Input: part model. Units: mm. Frame: model coordinates. A direction names the side the tool comes from. Coordinates: 2 decimals unless noted, no trailing zeros. Order: outer loops, then holes, each group sorted by start corner. A loop starts at its lowest first (then second) coordinate and runs counter-clockwise, first axis right, second up. Notation, with made-up numbers: M 7.25,84.25 L 38.25,84.25 A22 cw 38.25,110.25 Z; hole C 69.25,74 d11. An arc over 180 degrees is marked long. One line per item, written item: value.
```python
from build123d import *

# Parameters (mm, degrees)
SKETCH_1_R                   = 6.5
EXTRUDE_1_DEPTH              = 6.5
CUT_EXTRUDE_1_DEPTH          = 37.704904304
FILLET_2_R                   = 2.3
SWEEP_START                  = -22.062157242
SWEEP_2_DEPTH                = 13.492384883
CHAMFER_1_SIZE               = 0.5
FILLET_3_R                   = 3
HOLE_WIZARD_M2_1_D           = 2.4
HOLE_WIZARD_M2_1_DEPTH       = 8.5
HOLE_WIZARD_M2_1_CBORE_D     = 4.1
HOLE_WIZARD_M2_1_CBORE_DEPTH = 4.5
HOLE_WIZARD_M2_1_TIP         = 0.721032743
SKETCH_7_R                   = 1.05
CUT_EXTRUDE_2_DEPTH          = 6.5
CUT_EXTRUDE_3_DEPTH          = 4.5
CUT_EXTRUDE_4_DEPTH          = 2
PATTERN_CIRCULAR_1_COUNT     = 4


# Read off the part's stored shape, not the designer's step: ｶｯﾄ - ｽｲｰﾌﾟ2
with BuildPart() as part:
    # ｽｹｯﾁ1 → ﾎﾞｽ - 押し出し1 (new body)
    with BuildSketch(Plane(origin=(0, 0, 0), x_dir=(1, 0, 0), z_dir=(0, 1, 0))):
        with BuildLine():
            Line((-13.5, 13.5), (13.5, 13.5))
            Line((13.5, 13.5), (13.5, -24))
            Line((13.5, -24), (6.5, -24))
            Line((6.5, -24), (6.5, -21))
            ThreePointArc((6.5, -21), (0, -14.5), (-6.5, -21))
            Line((-6.5, -21), (-6.5, -24))
            Line((-6.5, -24), (-13.5, -24))
            Line((-13.5, -24), (-13.5, 13.5))
        make_face()
        with Locations(Location((0, 0, 0), (0, 0, 90))):
            Circle(SKETCH_1_R, mode=Mode.SUBTRACT)
    extrude(amount=EXTRUDE_1_DEPTH)

    # ｽｹｯﾁ2 → ｶｯﾄ - 押し出し1 (cut, through all)
    with BuildSketch(Plane(origin=(13.5, 0, 0), x_dir=(0, 0, -1), z_dir=(1, 0, 0))):
        Polygon((-24, 3), (-24, 6.5), (-13.5, 6.5), align=None)
    extrude(amount=-CUT_EXTRUDE_1_DEPTH, mode=Mode.SUBTRACT)

    # ﾌｨﾚｯﾄ2
    fillet_2_edges = [part.edges().sort_by_distance(p)[0] for p in [
        (-13.5, 3.25, -13.5),
        (13.5, 3.25, -13.5),
    ]]
    fillet(fillet_2_edges, radius=FILLET_2_R)

    # ｶｯﾄ - ｽｲｰﾌﾟ2 outline → ｶｯﾄ - ｽｲｰﾌﾟ2 (cut)
    with BuildSketch(Plane(origin=(0, 0, 0), x_dir=(1, 0, 0), z_dir=(0, 0.3162277660168393, -0.9486832980505134)).offset(SWEEP_START)):
        with BuildLine():
            Line((-13.5, -10.435516279), (-11.2, -10.435516279))
            add(Edge.make_bspline(
                [(-11.2, -10.435516279), (-12.547308807, -10.435516279), (-13.5, -10.134248871), (-13.5, -9.708192417)],
                knots=[0, 0, 0, 0, 1, 1, 1, 1], degree=3, weights=[1, 0.804737854, 0.804737854, 1]))
            Line((-13.5, -9.708192417), (-13.5, -10.435516279))
        make_face()
        with BuildLine():
            add(Edge.make_bspline(
                [(13.5, -9.708192417), (13.5, -10.134248871), (12.547308807, -10.435516279), (11.2, -10.435516279)],
                knots=[0, 0, 0, 0, 1, 1, 1, 1], degree=3, weights=[1, 0.804737854, 0.804737854, 1]))
            Line((11.2, -10.435516279), (13.5, -10.435516279))
            Line((13.5, -10.435516279), (13.5, -9.708192417))
        make_face()
    extrude(amount=SWEEP_2_DEPTH, mode=Mode.SUBTRACT)

    # 面取り1
    chamfer_1_edges = [part.edges().sort_by_distance(p)[0] for p in [
        (6.5, 1.5, 24),
        (-6.5, 1.5, 24),
    ]]
    chamfer(chamfer_1_edges, length=CHAMFER_1_SIZE)

    # ﾌｨﾚｯﾄ3
    # the kernel refuses this fillet: 3 mm, written as the material it takes off along each edge
    with BuildSketch(Plane(origin=(13.5, -7.5, 24), x_dir=(0, 0, -1), z_dir=(0, 1, 0)), Plane(origin=(-13.5, -7.5, 24), x_dir=(1, 0, 0), z_dir=(0, 1, 0))) as fillet_3_piece_1:
        with BuildLine():
            CenterArc((FILLET_3_R, FILLET_3_R), FILLET_3_R, 180, 90)
            Line((0, FILLET_3_R), (0, 0))
            Line((0, 0), (FILLET_3_R, 0))
        make_face()
    extrude(amount=17.233333302, mode=Mode.SUBTRACT)

    # M2 なべ頭ねじ用座ぐり穴1
    with Locations(Plane(origin=(0, 6.5, 0), x_dir=(1, 0, 0), z_dir=(0, 1, 0))):
        with Locations((-10.5, 0), (10.5, 0), (10.5, -21), (-10.5, -21)):
            CounterBoreHole(HOLE_WIZARD_M2_1_D / 2, HOLE_WIZARD_M2_1_CBORE_D / 2, HOLE_WIZARD_M2_1_CBORE_DEPTH, depth=HOLE_WIZARD_M2_1_DEPTH)
            with Locations((0, 0, -(HOLE_WIZARD_M2_1_DEPTH + HOLE_WIZARD_M2_1_TIP / 2))):  # 118° drill point
                Cone(0, HOLE_WIZARD_M2_1_D / 2, HOLE_WIZARD_M2_1_TIP, mode=Mode.SUBTRACT)

    # ｽｹｯﾁ7 → ｶｯﾄ - 押し出し2 (cut)
    with BuildSketch(Plane(origin=(0, 6.5, 0), x_dir=(1, 0, 0), z_dir=(0, 1, 0))):
        with Locations(Location((-10.5, 10.5, 0), (0, 0, 270))):
            Circle(SKETCH_7_R)
        with Locations(Location((10.5, 10.5, 0), (0, 0, 270))):
            Circle(SKETCH_7_R)
        with Locations(Location((-10.5, -10.5, 0), (0, 0, 270))):
            Circle(SKETCH_7_R)
        with Locations(Location((10.5, -10.5, 0), (0, 0, 270))):
            Circle(SKETCH_7_R)
    extrude(amount=-CUT_EXTRUDE_2_DEPTH, mode=Mode.SUBTRACT)

    # ｽｹｯﾁ8 → ｶｯﾄ - 押し出し3 (cut)
    with BuildSketch(Plane.XZ):
        Polygon((-8.213522103, 9.887340094), (-8.826182009, 12.173817991), (-11.112659906, 12.786477897), (-12.786477897, 11.112659906), (-12.173817991, 8.826182009), (-9.887340094, 8.213522103), align=None)
    cut_extrude_3 = extrude(amount=-CUT_EXTRUDE_3_DEPTH, mode=Mode.SUBTRACT)

    # ｽｹｯﾁ9 → ｶｯﾄ - 押し出し4 (cut)
    with BuildSketch(Plane.XZ):
        Polygon((-9.887340094, 8.213522103), (-4.230485845, 2.556667854), (-2.556667854, 4.230485845), (-8.213522103, 9.887340094), align=None)
    cut_extrude_4 = extrude(amount=-CUT_EXTRUDE_4_DEPTH, mode=Mode.SUBTRACT)

    # 円形ﾊﾟﾀｰﾝ1: ｶｯﾄ - 押し出し3, ｶｯﾄ - 押し出し4 ×4 about axis
    pattern_circular_1_axis = Axis((0, 0, 0), (0, 1, 0))
    add([cut_extrude_3.rotate(pattern_circular_1_axis, i * 360 / PATTERN_CIRCULAR_1_COUNT) for i in range(1, PATTERN_CIRCULAR_1_COUNT)], mode=Mode.SUBTRACT)
    add([cut_extrude_4.rotate(pattern_circular_1_axis, i * 360 / PATTERN_CIRCULAR_1_COUNT) for i in range(1, PATTERN_CIRCULAR_1_COUNT)], mode=Mode.SUBTRACT)


solid = part.part
```
(1) Draft query along X for faces 4 (the cylindrical face through (12.6, 1.59, 23.14)), 5 (the cylindrical face through (-11.054, 0.986, 22.065)), 6 (the cylindrical face through (-12.81, 3.3, -12.84)). Return one class per face: released by +X, released by -X, zero draft, split by the parting line, or undercut.
Data:
face 4: released by +X
face 5: undercut
face 6: released by -X
(2) First-contact query: pin 1 (2.5 mm diameter, centred on x = -10.5, z = 10.5, fed in from -Y); pin 2 (2 mm diameter, centred on y = 2.5, z = 22.5, fed in from -X); pin 3 (5.5 mm diameter, centred on x = 10.5, z = 21, fed in from +Y). Flat tips, straight axial feed; report the tip coordinate or a pass-through.
Data:
pin 1: stops at y = 4.5
pin 2: stops at x = -13.46
pin 3: stops at y = 4.92
(3) Ray query, line 1 (X direction, y = 0.65, z = 21); line 2 (X direction, y = 3.2, z = 21); line 3 (X direction, y = 5.45, z = 10.5). Return the intervals inside material, ascending. Write a range as from..to.
Data:
line 1: x = -13.5..-11.7, -9.3..-6.5, 6.5..9.3, 11.7..13.5
line 2: x = -13.5..-12.55, -8.45..-6.5, 6.5..8.45, 12.55..13.5
line 3: x = -13.5..-11.55, -9.45..9.45, 11.55..13.5
(4) Access query for faces 1 (the cylindrical face through (8.45, 4.28, -0.09)), 2 (the flat face through (11.9, 2.2, -12)), 3 (the flat face through (6.5, 2, 22)). Directions: +Z, -Z, +X, -X, +Y, -Y. A direction counts if a zero-diameter tool reaches every point of the face in a straight line with its end or side. Return the directions, or none.
Data:
face 1: +Y
face 2: -Y
face 3: +Z, +Y, -Y
(5) Cut plane B-B on x = 0. Output: boundary loops of the cut face in (y, z).
Data:
outline: M 0,-13.5 L 6.5,-13.5 L 6.5,-6.5 L 0,-6.5 Z; M 0,6.5 L 6.5,6.5 L 6.5,13.5 L 6.17,14.5 L 0,14.5 Z
(6) Cut plane C-C on z = -10.5. Output: boundary loops of the cut face in (x, y).
Data:
outline: M -13.5,0 L -12.62,0 L -12.62,4.5 L -11.55,4.5 L -11.55,6.5 L -13.5,6.5 Z; M -9.45,4.5 L -8.38,4.5 L -8.38,0 L 8.38,0 L 8.38,4.5 L 9.45,4.5 L 9.45,6.5 L -9.45,6.5 Z; M 11.55,4.5 L 12.62,4.5 L 12.62,0 L 13.5,0 L 13.5,6.5 L 11.55,6.5 Z
(7) Cut plane A-A on z = 0. Output: boundary loops of the cut face in (x, y).
Data:
outline: M -13.5,0 L -11.7,0 L -11.7,2 L -12.55,2 L -12.55,6.5 L -13.5,6.5 Z; M -9.3,0 L -6.5,0 L -6.5,6.5 L -8.45,6.5 L -8.45,2 L -9.3,2 Z; M 6.5,0 L 9.3,0 L 9.3,2 L 8.45,2 L 8.45,6.5 L 6.5,6.5 Z; M 11.7,0 L 13.5,0 L 13.5,6.5 L 12.55,6.5 L 12.55,2 L 11.7,2 Z
(8) Cut plane D-D on x = 7.5. Output: boundary loops of the cut face in (y, z).
Data:
outline: M 0,-13.5 L 6.5,-13.5 L 6.5,13.5 L 3,24 L 0,24 L 0,9.17 L 2,9.17 L 2,5.83 L 0,5.83 L 0,-5.83 L 2,-5.83 L 2,-9.17 L 0,-9.17 Z
